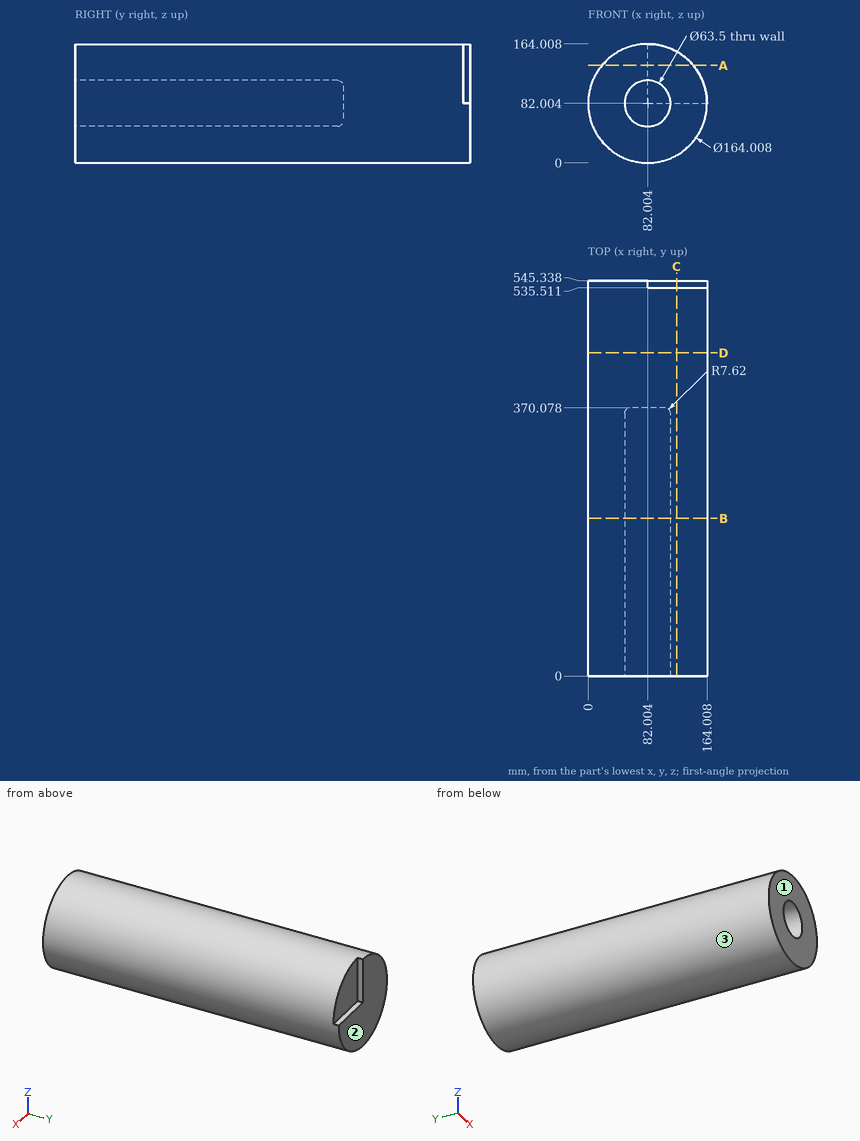
Check sheet for the drawn part. Datum: minimum x, y, z corner. Units: mm. Round coordinates to 2 decimals unless told otherwise and drop trailing zeros. Order: outer loops, then holes, each group sorted by start corner. A loop starts at its lowest first (then second) coordinate and runs counter-clockwise, first axis right, second up.
1. Section check C-C on x = 122. Record the cut outline in (y, z) (1 decimal), then the cut area to 3 significant figures.
Final values:
outline: (0, 10.4) - (545.3, 10.4) - (545.3, 82) - (535.5, 82) - (535.5, 153.6) - (0, 153.6) - close
area: 77,400 mm2
2. Go/stop test with flat-tipped pins: P1, Ø5, axis at y = 449, z = 134.5, coming from the +X side; P2, Ø3, axis at x = 116, z = 22, coming from the -Y side; P3, Ø3, axis at x = 121.5, y = 369.5, coming from the +Z side; P4, Ø2, axis at y = 466.5, z = 79, coming from the +X side. Record where each tip stops, or that it passes through.
Final values:
P1: stops at x = 147
P2: stops at y = 0
P3: stops at z = 154.67
P4: stops at x = 163.98
3. Release check for a two-part mould opening along Y. For the marked faces 1, 2 and 3 record: +Y half, -Y half, draft (parallel to the pull), parting line (faces both ways), or undercut.
Final values:
face 1: -Y half
face 2: +Y half
face 3: draft
4. Section check A-A on z = 134.5. Record the cut outline in (x, y), then the cut area to 3 significant figures.
Final values:
outline: (19.01, 0) - (145, 0) - (145, 535.51) - (82, 535.51) - (82, 545.34) - (19.01, 545.34) - close
area: 68,100 mm2
5. Thickness scan on L1, parallel to X at y = 328.5, z = 82; L2, parallel to X at y = 72.5, z = 79.5 (1 decimal); L3, parallel to Z at x = 86.5, y = 330.5. Record the ranges inside material, lowest first.
Final values:
L1: x = 0 to 50.25, 113.75 to 164.01
L2: x = 0 to 50.4, 113.7 to 164
L3: z = 0.12 to 50.57, 113.43 to 163.88
6. Section check D-D on y = 446. Record the cut outline in (x, z).
Final values:
outline: circle Ø164.01 at (82, 82)
7. Section check B-B on y = 217.5. Record the cut outline in (x, z).
Final values:
outline: circle Ø164.01 at (82, 82); hole circle Ø63.5 at (82, 82)
